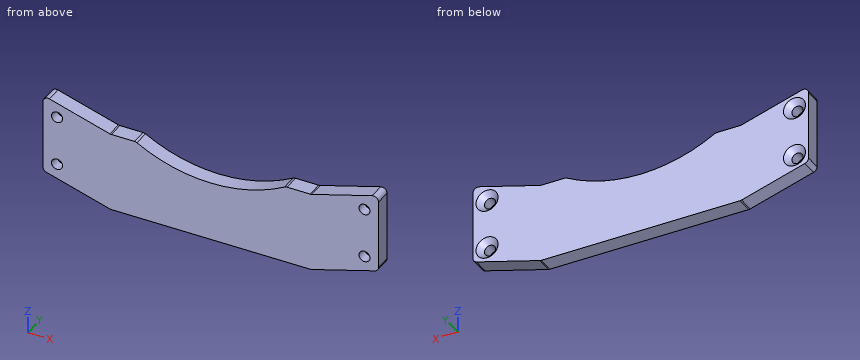
```python
from build123d import *

# Parameters (mm, degrees)
BOSS_EXTRUDE1_DEPTH                             = 3.175
CSK_FOR_M2_FLAT_HEAD_MACHINE_SCREW1_D           = 2.2
CSK_FOR_M2_FLAT_HEAD_MACHINE_SCREW1_CSINK_D     = 4.4
CSK_FOR_M2_FLAT_HEAD_MACHINE_SCREW1_CSINK_ANGLE = 90
SKETCH5_R                                       = 30
CUT_EXTRUDE2_DEPTH                              = 40.144994891
FILLET1_R                                       = 1


with BuildPart() as part:
    # Sketch1 → Boss-Extrude1 (new body)
    with BuildSketch(Plane(origin=(0, 0, 0), x_dir=(1, 0, 0), z_dir=(0, 1, 0))):
        Polygon((-33.5, 0), (-33.5, 16), (-20, 20), (0, 20), (0, 4), (-20, 4), align=None)
    extrude(amount=BOSS_EXTRUDE1_DEPTH)

    # CSK for M2 Flat Head Machine Screw1 (through all)
    with Locations(Plane(origin=(0, 3.175, 0), x_dir=(1, 0, 0), z_dir=(0, 1, 0))):
        with Locations((-30.7, 13.8), (-30.7, 3.8)):
            CounterSinkHole(CSK_FOR_M2_FLAT_HEAD_MACHINE_SCREW1_D / 2, CSK_FOR_M2_FLAT_HEAD_MACHINE_SCREW1_CSINK_D / 2, counter_sink_angle=CSK_FOR_M2_FLAT_HEAD_MACHINE_SCREW1_CSINK_ANGLE)

    # Mirror1: part across plane


with BuildPart() as part_1:
    add(part.part)
    add(part.part.mirror(Plane(origin=(0, 0, 0), x_dir=(0, 0, 1), z_dir=(1, 0, 0))))

    # Sketch5 → Cut-Extrude2 (cut, through all)
    with BuildSketch(Plane(origin=(0, 3.175, 0), x_dir=(1, 0, 0), z_dir=(0, 1, 0))):
        with Locations((0, -22)):
            Circle(SKETCH5_R)
    extrude(amount=-CUT_EXTRUDE2_DEPTH, mode=Mode.SUBTRACT)

    # Fillet1
    fillet1_edges = [part_1.edges().sort_by_distance(p)[0] for p in [
        (-20, 1.5875, -4),
        (-33.5, 1.5875, 0),
        (-33.5, 1.5875, -16),
        (-20, 1.5875, -20),
        (20, 1.5875, -20),
        (33.5, 1.5875, -16),
        (33.5, 1.5875, 0),
        (20, 1.5875, -4),
        (-14.966629547, 1.5875, -4),
        (14.966629547, 1.5875, -4),
    ]]
    fillet(fillet1_edges, radius=FILLET1_R)


solid = part_1.part
```
The model under review builds one solid part; all positions refer to its coordinate system, in mm. Round coordinates to 2 decimals unless told otherwise and drop trailing zeros. Loops run counter-clockwise (first coordinate to the right, second up) from the corner with the lowest first, then second, coordinate; pieces in that order, holes last.
Item 1: Clearance check with a flat-ended pin moving along its axis: pin 1 Ø2.5 at (x, z) = (-30.7, -13.8) entering from +Y (3 decimals). State where the tip first meets the part, or that it passes through.
Determined:
pin 1: stops at y = 2.225
Item 2: Take a section at C-C (x = 30.7). Write out the cut boundary in (y, z) (3 decimals).
Determined:
outline: (0, -16.83) - (3.175, -16.83) - (3.175, -16) - (2.075, -14.9) - (0, -14.9) - close; (0, -12.7) - (2.075, -12.7) - (3.175, -11.6) - (3.175, -6) - (2.075, -4.9) - (0, -4.9) - close; (0, -2.7) - (2.075, -2.7) - (3.175, -1.6) - (3.175, -0.83) - (0, -0.83) - close
Item 3: Take a section at B-B (z = -13.8). Write out the cut boundary in (x, y) (3 decimals).
Determined:
outline: (-33.5, 0) - (-31.8, 0) - (-31.8, 2.075) - (-32.9, 3.175) - (-33.5, 3.175) - close; (-29.6, 0) - (29.6, 0) - (29.6, 2.075) - (28.5, 3.175) - (-28.5, 3.175) - (-29.6, 2.075) - close; (31.8, 0) - (33.5, 0) - (33.5, 3.175) - (32.9, 3.175) - (31.8, 2.075) - close
Item 4: Take a section at A-A (y = 1). Write out the cut boundary in (x, z), then the cut area to 3 significant figures.
Determined:
outline: (-33.5, -15.25) arc R1 ccw to (-32.78, -16.21) - (-20.14, -19.96) arc R1 ccw to (-19.85, -20) - (19.85, -20) arc R1 ccw to (20.14, -19.96) - (32.78, -16.21) arc R1 ccw to (33.5, -15.25) - (33.5, -1.34) arc R1 ccw to (32.22, -0.38) - (20.14, -3.96) arc R1 cw to (19.85, -4) - (15.23, -4) arc R1 ccw to (14.74, -4.13) arc R30 cw to (-14.74, -4.13) arc R1 ccw to (-15.23, -4) - (-19.85, -4) arc R1 cw to (-20.14, -3.96) - (-32.22, -0.38) arc R1 ccw to (-33.5, -1.34) - close; hole circle Ø2.2 at (-30.7, -13.8); hole circle Ø2.2 at (-30.7, -3.8); hole circle Ø2.2 at (30.7, -13.8); hole circle Ø2.2 at (30.7, -3.8)
area: 975 mm2
Item 5: For line 1 (X direction, y = 1.6, z = -13.8); line 2 (Z direction, x = 30.7, y = 1.65); line 3 (X direction, y = 0.25, z = -14.25), list the stretches that pass through material, from the lowest coordinate up.
Determined:
line 1: x = -33.5 to -31.8, -29.6 to 29.6, 31.8 to 33.5
line 2: z = -16.83 to -14.9, -12.7 to -4.9, -2.7 to -0.83
line 3: x = -33.5 to -31.7, -29.7 to 29.7, 31.7 to 33.5
